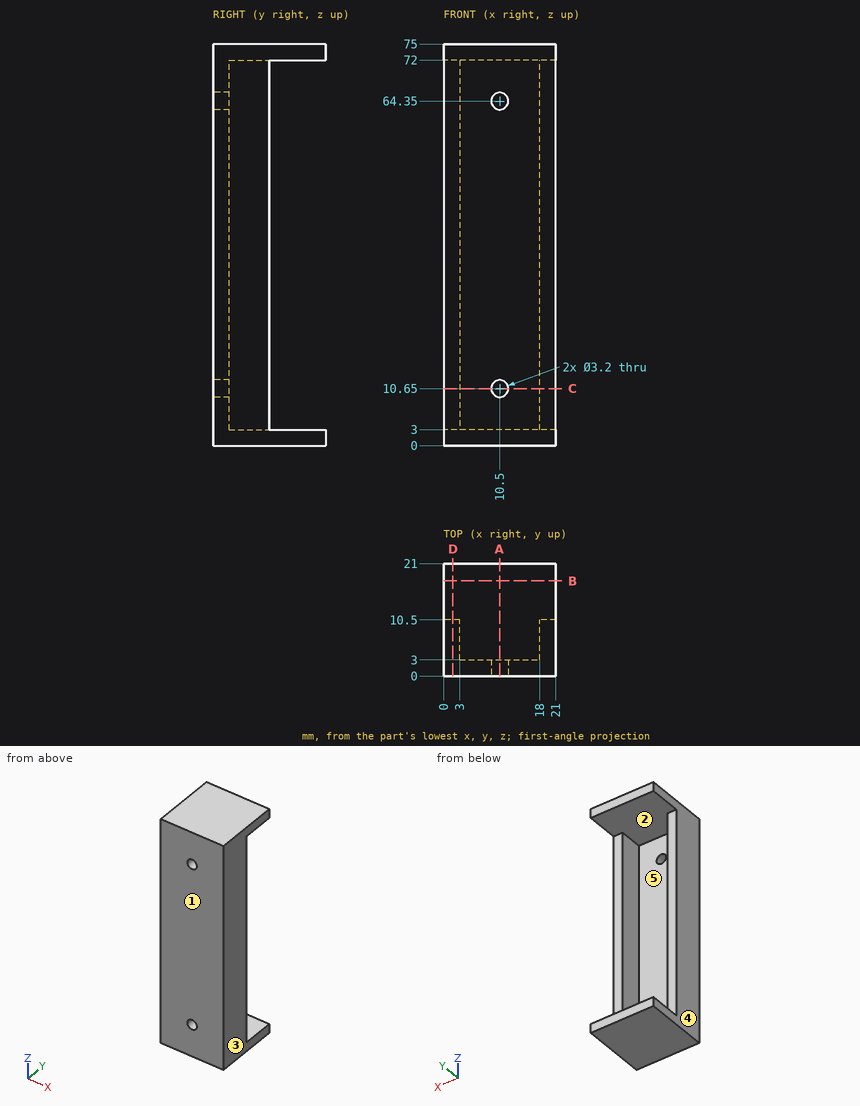
Design review of the part shown in the three views and the two pictorial views. Dimensions are in mm from the part's minimum x, y and z. A direction names the side the tool comes from. Coordinates: 2 decimals unless noted, no trailing zeros. Order: outer loops, then holes, each group sorted by start corner. A loop starts at its lowest first (then second) coordinate and runs counter-clockwise, first axis right, second up.
1) Clearance check with flat-ended pins moving along their axes: pin 1 (2.5 mm diameter, centred on x = 10.5, z = 10.65, fed in from -Y); pin 2 (1.5 mm diameter, centred on x = 3, z = 37.5, fed in from +Y). State where each tip first meets the part, or that it passes through.
2) Take a section at D-D, the plane x = 1.75. Give the boundary of the cut face in (y, z).
3) Take a section at A-A, the plane x = 10.5. Give the boundary of the cut face in (y, z), and give its area (3 significant figures).
4) Mouldability with a two-part tool opening along X and no side actions: class the marked faces 1, 2 and 3 as +X half, -X half, draft (parallel to the pull), parting line (faces both ways), or undercut.
5) For the marked faces 4 and 5, list the 3-axis set-ups (+Z, -Z, +X, -X, +Y, -Y) from which the entire face can be reached by the end or side of a thin tool; tool diameter is ignored.
6) Wall thickness on line 1 along Z through (x, y) = (10.5, 1.9); line 2 along X through (y, z) = (7.25, 31); line 3 along Z through (x, y) = (14.75, 9.25): over which ranges is each line inside the solid? List them lowest first.
7) Take a section at C-C, the plane z = 10.65. Give the boundary of the cut face in (x, y).
8) Take a section at B-B, the plane y = 17.75. Give the boundary of the cut face in (x, z).
Returned:
1. pin 1: passes through
1. pin 2: stops at y = 10.5
2. outline: (0, 0) - (21, 0) - (21, 3) - (10.5, 3) - (10.5, 72) - (21, 72) - (21, 75) - (0, 75) - close
3. outline: (0, 0) - (21, 0) - (21, 3) - (3, 3) - (3, 9.05) - (0, 9.05) - close; (0, 12.25) - (3, 12.25) - (3, 62.75) - (0, 62.75) - close; (0, 65.95) - (3, 65.95) - (3, 72) - (21, 72) - (21, 75) - (0, 75) - close
3. area: 314 mm2
4. face 1: draft
4. face 2: undercut
4. face 3: +X half
5. face 4: +Z, -Z, -X, +Y, -Y
5. face 5: +Y
6. line 1: z = 0 to 9.05, 12.25 to 62.75, 65.95 to 75
6. line 2: x = 0 to 3, 18 to 21
6. line 3: z = 0 to 3, 72 to 75
7. outline: (0, 0) - (8.9, 0) - (8.9, 3) - (3, 3) - (3, 10.5) - (0, 10.5) - close; (12.1, 0) - (21, 0) - (21, 10.5) - (18, 10.5) - (18, 3) - (12.1, 3) - close
8. outline: (0, 0) - (21, 0) - (21, 3) - (0, 3) - close; (0, 72) - (21, 72) - (21, 75) - (0, 75) - close
